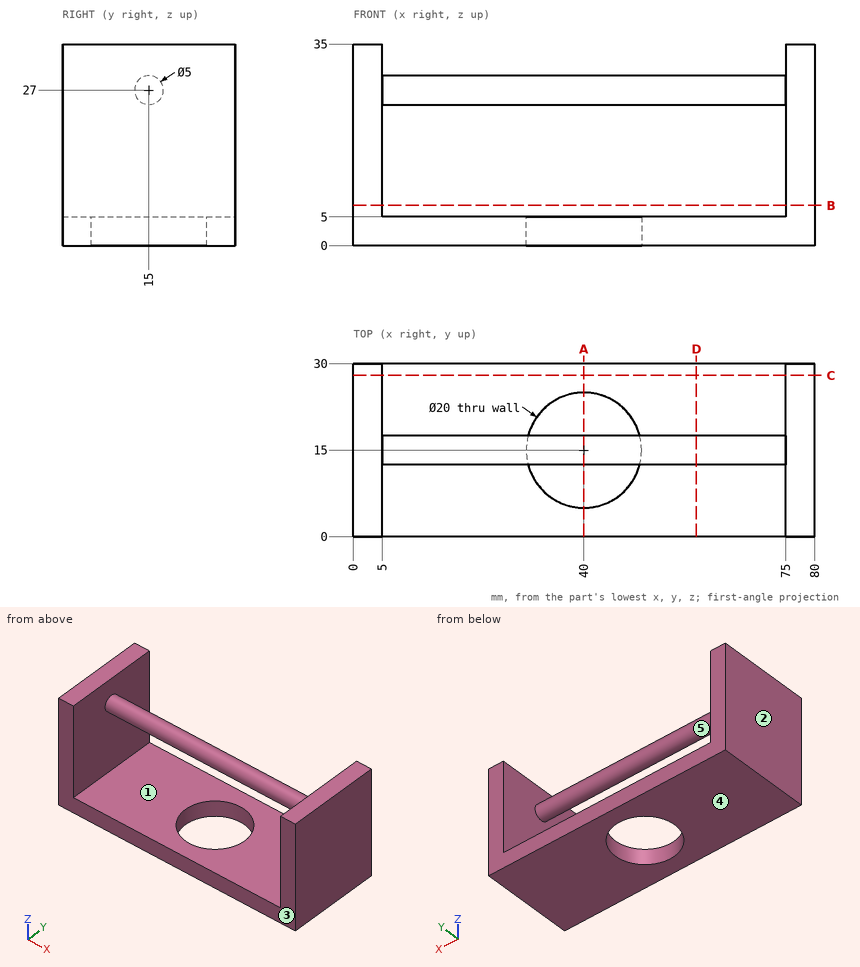
Job drawing, mm, ordinate dimensions from the low corner. One solid piece. A direction names the side the tool comes from. Round coordinates to 2 decimals unless told otherwise and drop trailing zeros. Loops run counter-clockwise (first coordinate to the right, second up) from the corner with the lowest first, then second, coordinate; pieces in that order, holes last. Notation, with made-up numbers: (43.25, 89.25) -> (47.25, 89.25) arc R28 ccw to (47.25, 123.25) -> close; hole circle Ø7 at (8, -12). An arc over 180 degrees is marked (long way). Use CSV: the item, a comma, the result in double quotes. Start each with the question number.
Q1. Saw through at D-D on x = 59.5. Give the cut face in (y, z), and give its area (3 significant figures).
Q2. Mould opens along X. For the marked faces 1, 2 and 3 say: +X half, -X half, draft (parallel to the pull), parting line (faces both ways), or undercut.
Q3. Saw through at B-B on z = 7. Give the cut face in (x, y), and give its area (3 significant figures).
Q4. Which spindle directions (+Z, -Z, +X, -X, +Y, -Y) get a long thin tool onto all of the face, cutting with end or side? Do the marked faces 4 and 5. Say none if no direction does.
Q5. Drill centre lines: L1, parallel to X at y = 26.75, z = 16; L2, parallel to Y at x = 40, z = 1; L3, parallel to X at y = 15.5, z = 2. Where is each one in solid material? Low to high.
Q6. Saw through at C-C on y = 28. Give the cut face in (x, z), and give its area (3 significant figures).
Q7. Flat gauge pins, fed straight in: pin 1 Ø2 at (y, z) = (20, 30.5) entering from -X; pin 2 Ø15 at (x, y) = (45.5, 16) entering from +Z. Where does each tip first touch, or does it go through?
Q8. Saw through at A-A on x = 40. Give the cut face in (y, z), and give its area (3 significant figures).
Solutions:
1,outline,"(0, 0) -> (30, 0) -> (30, 5) -> (0, 5) -> close; circle Ø5 at (15, 27)"
1,area,"170 mm^2"
2,face 1,"undercut"
2,face 2,"-X half"
2,face 3,"draft"
3,outline,"(0, 0) -> (5, 0) -> (5, 30) -> (0, 30) -> close; (75, 0) -> (80, 0) -> (80, 30) -> (75, 30) -> close"
3,area,"300 mm^2"
4,face 4,"-Z, +X, -X, +Y, -Y"
4,face 5,"none"
5,L1,"x = 0 to 5, 75 to 80"
5,L2,"y = 0 to 5, 25 to 30"
5,L3,"x = 0 to 30.01, 49.99 to 80"
6,outline,"(0, 0) -> (80, 0) -> (80, 35) -> (75, 35) -> (75, 5) -> (5, 5) -> (5, 35) -> (0, 35) -> close"
6,area,"700 mm^2"
7,pin 1,"stops at x = 0"
7,pin 2,"stops at z = 29.5"
8,outline,"(0, 0) -> (5, 0) -> (5, 5) -> (0, 5) -> close; circle Ø5 at (15, 27); (25, 0) -> (30, 0) -> (30, 5) -> (25, 5) -> close"
8,area,"69.6 mm^2"
